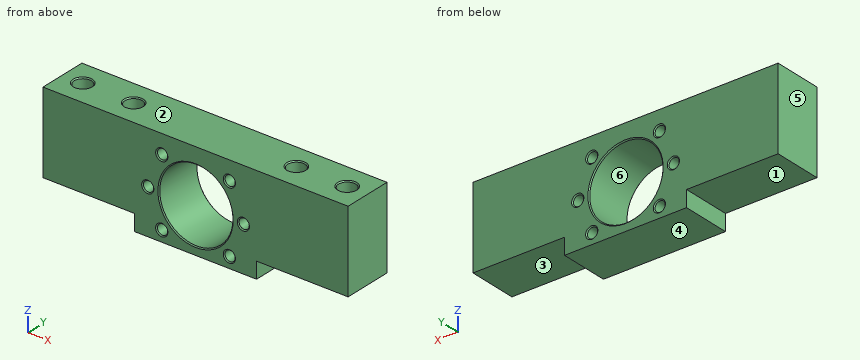
from build123d import *

# Parameters (mm, degrees)
F0_R     = 18
F1_DEPTH = 24
F2_R     = 2.5
F3_DEPTH = 25
F4_R     = 4.25
F5_DEPTH = 35
F6_SIZE  = 4.25
F7_SIZE  = 0.5


with BuildPart() as f1:
    # F0 (on Front) → F1 (new body)
    with BuildSketch(Plane.XZ):
        Polygon((-30, -22), (30, -22), (30, -14), (75, -14), (75, 26), (-75, 26), (-75, -14), (-30, -14), align=None)
        Circle(F0_R, mode=Mode.SUBTRACT)
    extrude(amount=F1_DEPTH)

    # F2 (on face) → F3 (cut)
    with BuildSketch(Plane.XZ.offset(24)):
        with Locations((-23.5, 0)):
            Circle(F2_R)
        with Locations((-16.617009, -16.617009)):
            Circle(F2_R)
        with Locations((16.617009, -16.617009)):
            Circle(F2_R)
        with Locations((23.5, 0)):
            Circle(F2_R)
        with Locations((16.617009, 16.617009)):
            Circle(F2_R)
        with Locations((-16.617009, 16.617009)):
            Circle(F2_R)
    extrude(amount=-F3_DEPTH, mode=Mode.SUBTRACT)

    # F4 (on face) → F5 (cut)
    with BuildSketch(Plane.XY.offset(26)):
        with Locations((-65, -12)):
            Circle(F4_R)
        with Locations((-40, -12)):
            Circle(F4_R)
        with Locations((65, -12)):
            Circle(F4_R)
        with Locations((40, -12)):
            Circle(F4_R)
    extrude(amount=-F5_DEPTH, mode=Mode.SUBTRACT)

    # F6
    f6_edges = [f1.edges().sort_by_distance(p)[0] for p in [
        (-69.25, -12, -9),
        (-44.25, -12, -9),
        (35.75, -12, -9),
        (60.75, -12, -9),
    ]]
    chamfer(f6_edges, length=F6_SIZE)

    # F7
    f7_edges = [f1.edges().sort_by_distance(p)[0] for p in [
        (-69.25, -12, 26),
        (-44.25, -12, 26),
        (35.75, -12, 26),
        (60.75, -12, 26),
        (18, -12, 0),
        (-18, 0, 0),
        (-18, -24, 0),
        (-26, -24, 0),
        (-21, -12, 0),
        (-26, 0, 0),
        (-19.117009, -24, 16.617009),
        (-14.117009, -12, 16.617009),
        (-19.117009, 0, 16.617009),
        (-19.117009, -24, -16.617009),
        (-14.117009, -12, -16.617009),
        (-19.117009, 0, -16.617009),
        (14.117009, -24, -16.617009),
        (19.117009, -12, -16.617009),
        (14.117009, 0, -16.617009),
        (21, -24, 0),
        (26, -12, 0),
        (21, 0, 0),
        (14.117009, -24, 16.617009),
        (19.117009, -12, 16.617009),
        (14.117009, 0, 16.617009),
    ]]
    chamfer(f7_edges, length=F7_SIZE)


solid = f1.part
Could you check a few things on this model? Use its own coordinates, in mm. Face numbers are marked on the shaded views. A direction names the side the tool comes from. Coordinates: 2 decimals unless noted, no trailing zeros. Write each loop counter-clockwise with the first axis right and the second up, starting at its lowest first coordinate (ties: lowest second). Pieces come first, ordered by that corner, then holes. Notation, with made-up numbers: (86, 42) - (127, 42) arc R9 ccw to (127, 53) - close; hole circle Ø9 at (63, 57). An arc over 180 degrees is marked (long way). Write item = value, one per line.
1) We'd pull the mould along X, two halves only. Please class the marked faces 4, 5 and 6: +X half, -X half, draft (parallel to the pull), parting line (faces both ways), or undercut.
Result set:
face_4 = draft
face_5 = -X half
face_6 = undercut
2) Suppose I cut it at A-A on z = 0. State how many separate pieces and enclosed holes the cut face has, plus the area to 3 significant figures.
Result set:
separate_pieces = 4
enclosed_holes = 4
area = 2,270 mm2
3) Suppose I cut it at B-B on x = -23.5. Please give me the cut outline in (y, z), plus the area to 3 significant figures.
Result set:
outline = (-24, -22) - (0, -22) - (0, -3) - (-0.5, -2.5) - (-23.5, -2.5) - (-24, -3) - close; (-24, 3) - (-23.5, 2.5) - (-0.5, 2.5) - (0, 3) - (0, 26) - (-24, 26) - close
area = 1,030 mm2
4) Please list where these lines run through material, in increasing order: line 1 (Y direction, x = -65, z = 6); line 2 (X direction, y = -6.75, z = 1.5); line 3 (X direction, y = -19.5, z = 6.5). Write a range as [from, to].
Result set:
line_1 = [-24, -16.25], [-7.75, 0]
line_2 = [-75, -25.5], [-21.5, -17.94], [17.94, 21.5], [25.5, 75]
line_3 = [-75, -16.79], [16.79, 75]
5) Will these pins go through, and if not, where does the flat tip stop? pin 1 Ø7.5 at (x, y) = (-40, -12) entering from +Z; pin 2 Ø2.5 at (y, z) = (-12, -18.5) entering from -X; pin 3 Ø5 at (x, y) = (65, -12) entering from -Z.
Result set:
pin_1 = -5.25
pin_2 = -30
pin_3 = -14
6) Suppose I cut it at C-C on y = -21. Please give me the cut outline in (x, z), plus the area to 3 significant figures.
Result set:
outline = (-75, -14) - (-30, -14) - (-30, -22) - (30, -22) - (30, -14) - (75, -14) - (75, 26) - (-75, 26) - close; hole circle Ø5 at (-23.5, 0); hole circle Ø5 at (-16.62, -16.62); hole circle Ø5 at (-16.62, 16.62); hole circle Ø36 at (0, 0); hole circle Ø5 at (16.62, -16.62); hole circle Ø5 at (16.62, 16.62); hole circle Ø5 at (23.5, 0)
area = 5,340 mm2
7) For the marked faces 1, 2 and 3, which set-ups out of +Z, -Z, +X, -X, +Y, -Y let a thin tool reach every point of the face, with its end or its side?
Result set:
face_1 = -Z, -X, +Y, -Y
face_2 = +Z, +X, -X, +Y, -Y
face_3 = -Z, +X, +Y, -Y
